Print and shaded views of the part. All mm, measured from the part's lowest x, y and z. A direction names the side the tool comes from. Round coordinates to 2 decimals unless told otherwise and drop trailing zeros. Order: outer loops, then holes, each group sorted by start corner. A loop starts at its lowest first (then second) coordinate and runs counter-clockwise, first axis right, second up. Notation, with made-up numbers: (1.25, 46) - (39.25, 46) arc R3 ccw to (39.25, 51) - close; hole circle Ø1 at (81, 86.5). An arc over 180 degrees is marked (long way). Return JSON: item names as keys, results as strings. Group by question number.
Item 1: Saw through at B-B on x = 12.5. List the corners of the cut face in (y, z).
Item 2: Probe probe 1 along X at (y, z) = (55, 26); probe 2 along Y at (x, z) = (19.5, 21); probe 3 along Z at (x, y) = (12.5, 55.25). List the from-to ranges inside material, lowest first.
Item 3: Saw through at D-D on z = 6. List the corners of the cut face in (x, y), and give its area (3 significant figures).
Item 4: Saw through at C-C on y = 51. List the corners of the cut face in (x, z), and give its area (3 significant figures).
Item 5: Saw through at A-A on x = 64. List the corners of the cut face in (y, z).
Item 6: Two-plate mould, pull along Y, no slides. Class the marked faces 1, 2, 3 and 4: released by +Y, released by -Y, zero draft, split by the parting line, or undercut.
Item 7: Drop flat-ended pins along their axis: pin 1 (3 mm diameter, centred on y = 40.5, z = 28, fed in from +X); pin 2 (3 mm diameter, centred on y = 7.5, z = 14, fed in from +X). Give the stop position or say it passes through.
Item 8: Tool access for the marked faces 5 and 6: list every direction of +Z, -Z, +X, -X, +Y, -Y with a clear straight run to the whole face (end or side of a thin tool).
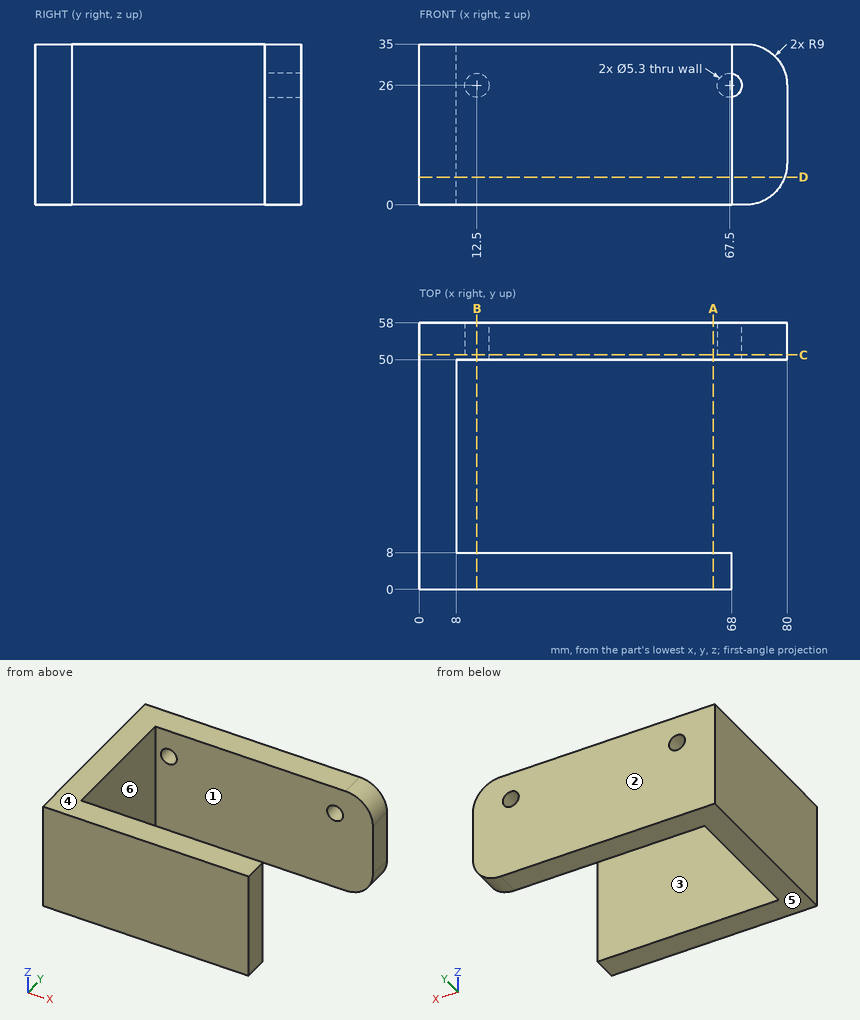
Filled in:
{
 "1": {"outline": "(0, 0) - (8, 0) - (8, 35) - (0, 35) - close; (50, 0) - (58, 0) - (58, 23.35) - (50, 23.35) - close; (50, 28.65) - (58, 28.65) - (58, 35) - (50, 35) - close"},
 "2": {"probe 1": "x = 0 to 9.85, 15.15 to 64.85, 70.15 to 80", "probe 2": "y = 0 to 8, 50 to 58", "probe 3": "z = 0 to 23.35, 28.65 to 35"},
 "3": {"outline": "(0, 0) - (68, 0) - (68, 8) - (8, 8) - (8, 50) - (79.49, 50) - (79.49, 58) - (0, 58) - close", "area": "1,520 mm^2"},
 "4": {"outline": "(0, 0) - (71, 0) arc R9 ccw to (80, 9) - (80, 26) arc R9 ccw to (71, 35) - (0, 35) - close; hole circle Ø5.3 at (12.5, 26); hole circle Ø5.3 at (67.5, 26)", "area": "2,720 mm^2"},
 "5": {"outline": "(0, 0) - (8, 0) - (8, 35) - (0, 35) - close; (50, 0) - (58, 0) - (58, 35) - (50, 35) - close"},
 "6": {"face 1": "undercut", "face 2": "released by +Y", "face 3": "undercut", "face 4": "zero draft"},
 "7": {"pin 1": "stops at x = 8", "pin 2": "stops at x = 68"},
 "8": {"face 5": "-Z, +X, -X, +Y, -Y", "face 6": "+Z, -Z, +X"}
}
